Here's the drawing with two shaded views (mm, measured from the low corner). I have some questions. Give positions to 0.01 mm unless a question says otherwise; leave off trailing zeros. Loops run counter-clockwise (first coordinate to the right, second up) from the corner with the lowest first, then second, coordinate; pieces in that order, holes last.
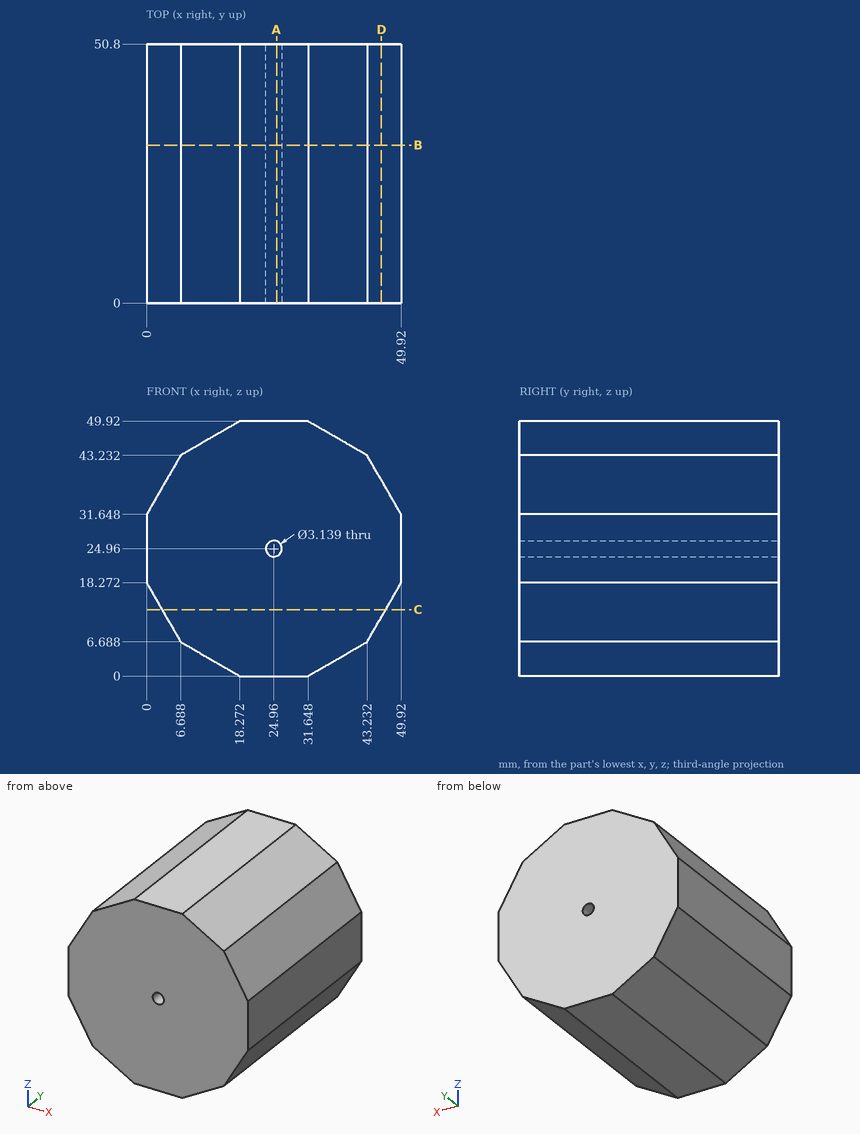
(1) Suppose I cut it at B-B on y = 31. List the corners of the cut face in (x, z) for me, plus the area to 3 significant figures.
Returned:
outline: (0, 18.27) - (6.69, 6.69) - (18.27, 0) - (31.65, 0) - (43.23, 6.69) - (49.92, 18.27) - (49.92, 31.65) - (43.23, 43.23) - (31.65, 49.92) - (18.27, 49.92) - (6.69, 43.23) - (0, 31.65) - close; hole circle Ø3.14 at (24.96, 24.96)
area: 2,000 mm2
(2) Will these pins go through, and if not, where does the flat tip stop? P1, Ø10, axis at y = 27.5, z = 9, coming from the -X side (1 decimal); P2, Ø1, axis at x = 6, y = 28, coming from the +Z side (1 decimal); P3, Ø2, axis at x = 35.5, y = 45.5, coming from the -Z side.
Returned:
P1: stops at x = 2.5
P2: stops at z = 42.9
P3: stops at z = 1.65
(3) Suppose I cut it at D-D on x = 46. List the corners of the cut face in (y, z) for me, plus the area to 3 significant figures.
Returned:
outline: (0, 11.48) - (50.8, 11.48) - (50.8, 38.44) - (0, 38.44) - close
area: 1,370 mm2
(4) Suppose I cut it at A-A on x = 25.5. List the corners of the cut face in (y, z) for me.
Returned:
outline: (0, 0) - (50.8, 0) - (50.8, 23.49) - (0, 23.49) - close; (0, 26.43) - (50.8, 26.43) - (50.8, 49.92) - (0, 49.92) - close
(5) Suppose I cut it at C-C on z = 13. List the corners of the cut face in (x, y) for me (1 decimal).
Returned:
outline: (3, 0) - (46.9, 0) - (46.9, 50.8) - (3, 50.8) - close
(6) Please list where these lines run through material, in increasing order: probe 1 along X at (y, z) = (5.5, 35) (1 decimal); probe 2 along X at (y, z) = (31, 33); probe 3 along Z at (x, y) = (13, 15.5) (1 decimal).
Returned:
probe 1: x = 1.9 to 48
probe 2: x = 0.78 to 49.14
probe 3: z = 3 to 46.9
